Design review of the part built by this model. Coordinates are the model's own, in mm. A direction names the side the tool comes from. Coordinates: 2 decimals unless noted, no trailing zeros. Write each loop counter-clockwise with the first axis right and the second up, starting at its lowest first coordinate (ties: lowest second). Pieces come first, ordered by that corner, then holes.
Q1. To check wall thickness, follow probe 1 along Y at (x, z) = (0, 1.75); probe 2 along X at (y, z) = (0, -76.5); probe 3 along Y at (x, z) = (0, 3.5). State the ranges of each line that lie inside material, in increasing order.
Q2. Add section B-B, the plane z = -12. Give the boundary of the cut face in (x, y), plus the area to 3 significant figures.
Q3. Add section A-A, the plane z = -60. Give the boundary of the cut face in (x, y), plus the area to 3 significant figures.
Q4. Clearance check with flat-ended pins moving along their axes: pin 1 Ø0.5 at (x, y) = (0.5, 0) entering from -Z; pin 2 Ø2 at (x, y) = (0, 0) entering from +Z; pin 3 Ø4.5 at (x, y) = (-0.5, 9.5) entering from +Z. State where each tip first meets the part, or that it passes through.
Q5. The part is to be moulded in two halves that separate along Y. For faces 1 (the face through (0.8, 1, -73)), 2 (the face through (-5.417, -1.203, -19.72)), 3 (the face through (0.48, -0.76, -74.48)), 4 (the face through (-3.854, 8.873, 1.479)), say which applies: +Y half, -Y half, draft (parallel to the pull), parting line (faces both ways), or undercut.
Q6. Machinability: for faces 5 (the face through (-1, 9.3, 3)), 6 (the face through (1.29, 2.024, 3.098)), 7 (the face through (0, 1.4, -76.8)), 8 (the face through (0, -2, -59)), which of the approach directions +Z, -Z, +X, -X, +Y, -Y give a long, thin tool a straight path to every point of the face, cutting with its end or side? Answer none if there is none.
from build123d import *

# Parameters (mm, degrees)
F0_R      = 0.9
F1_DEPTH  = 3
F5_W      = 1.6
F5_H      = 8
F6_DEPTH  = 9
F7_R      = 0.9
F8_DEPTH  = 11.2
F9_R      = 2.4
F10_DEPTH = 14


with BuildPart() as f1:
    # F0 (on Top) → F1 (new body)
    with BuildSketch(Plane.XY):
        with BuildLine():
            Line((-1.414214, 11.313708), (-6.363961, 6.363961))
            ThreePointArc((-6.363961, 6.363961), (0, -9), (6.363961, 6.363961))
            Line((6.363961, 6.363961), (1.414214, 11.313708))
            ThreePointArc((1.414214, 11.313708), (0, 11.899495), (-1.414214, 11.313708))
        make_face()
        with Locations((0, 9.899495)):
            Circle(F0_R, mode=Mode.SUBTRACT)
    extrude(amount=F1_DEPTH)

    # F2 (on Right) → F3 (revolve)
    with BuildSketch(Plane.YZ):
        with BuildLine():
            Line((0, 10), (0, 3))
            Line((0, 3), (9, 3))
            ThreePointArc((9, 3), (7.163441, 7.497235), (3, 10))
            Line((3, 10), (0, 10))
        make_face()
        with BuildLine():
            Line((9, 0), (0, 0))
            Line((0, 0), (0, -80))
            Line((0, -80), (1, -80))
            ThreePointArc((1, -80), (1.707107, -79.707107), (2, -79))
            Line((2, -79), (2, -40))
            Line((2, -40), (9, 0))
        make_face()
    revolve(axis=Axis((0, 0, -40), (0, 0, -1)))

    # F5 (on offset) → F6 (cut)
    with BuildSketch(Plane.XZ.offset(-9)):
        with Locations((0, -72.8)):
            Rectangle(F5_W, F5_H)
    extrude(amount=F6_DEPTH, mode=Mode.SUBTRACT)

    # F7 (on face) → F8 (cut)
    with BuildSketch(Plane(origin=(0, 0, -80), x_dir=(1, 0, 0), z_dir=(0, 0, -1))):
        Circle(F7_R)
    extrude(amount=-F8_DEPTH, mode=Mode.SUBTRACT)

    # F9 (on face) → F10 (cut)
    with BuildSketch(Plane.XY.offset(10)):
        Circle(F9_R)
    extrude(amount=-F10_DEPTH, mode=Mode.SUBTRACT)


solid = f1.part
Here are the results:
1. probe 1: y = -9 to -2.4, 2.4 to 9, 10.8 to 11.9
1. probe 2: x = -2 to -0.9, 0.9 to 2
1. probe 3: y = -8.95 to -2.4, 2.4 to 8.95
2. outline: circle Ø13.8 at (0, 0)
2. area: 150 mm2
3. outline: circle Ø4 at (0, 0)
3. area: 12.6 mm2
4. pin 1: stops at z = -68.8
4. pin 2: stops at z = -4
4. pin 3: stops at z = 7.38
5. face 1: draft
5. face 2: parting line
5. face 3: undercut
5. face 4: +Y half
6. face 5: +Z, +Y
6. face 6: +Z
6. face 7: +Y
6. face 8: -Z
